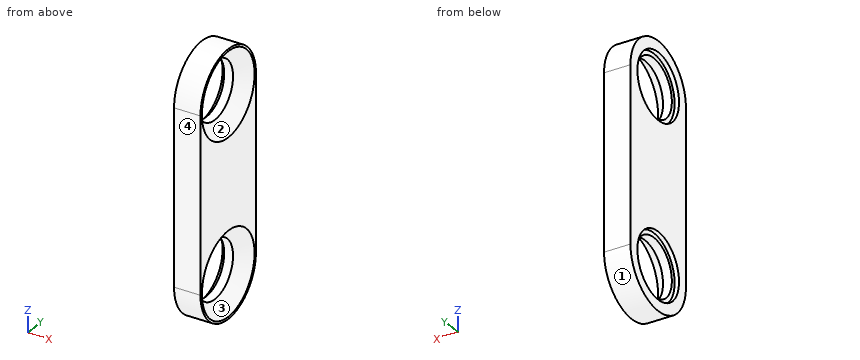
Autodesk Inventor part; units mm, degrees
ref_plane "YZ Plane" through (0, 0, 0) normal (1, 0, 0) x (0, 1, 0)
ref_plane "XZ Plane" through (0, 0, 0) normal (0, 1, 0) x (-1, 0, 0)
ref_plane "XY Plane" through (0, 0, 0) normal (0, 0, 1) x (1, 0, 0)
sketch "Boceto1" plane through (0, 0, 0) normal (1, 0, 0) x (0, 1, 0)
  line L0 (0, 0) -> (0, 19.75)
  circle A0 centre (0, 19.75) radius 5
  circle A1 centre (0, 0) radius 5
  line L1 (5, 0) -> (5, 19.75)
  line L2 (-5, 0) -> (-5, 19.75)
  circle A2 centre (0, 19.75) radius 3.25
  circle A3 centre (0, 0) radius 3.25
  dimension "d0" = 19.75
  dimension "d1" = 10
  dimension "d2" = 10
  dimension "d5" = 6.5
  dimension "d6" = 6.5
extrude "Extrusión1" add sketch "Boceto1" along normal mid plane 3
sketch "Boceto2" plane through (-1.5, 0, 0) normal (-1, 0, 0) x (0, 0, 1)
  circle A0 centre (0, 0) radius 3.75
  line L0 (0, 0) -> (19.75, 0)
  circle A1 centre (19.75, 0) radius 3.75
  dimension "d7" = 7.5
  dimension "d8" = 19.75
  dimension "d9" = 7.5
extrude "Extrusión2" cut sketch "Boceto2" against normal blind 0.5
chamfer "Chaflán1" distance 1.5 angle 45 2 edges at (1.5, -3.25, 19.75) (1.5, -3.25, 0)
equation "\"d0\" = m2_r3"
equation "\"d1\" = width_r3"
equation "\"d2\" = width_r3"
equation "\"d5\" = sj_diam_shaft + 0.5 * offset"
equation "\"d6\" = sj_diam_shaft + 0.5 * offset"
equation "\"d3\" = t_thikness"
equation "\"d7\" = sj_head_D + 0.5 * offset"
equation "\"d8\" = m2_r3"
equation "\"d9\" = sj_head_D + 0.5 * offset"
equation "\"d10\" = 0.5 * offset"
equation "\"offset\" = 1"
equation "\"m2_r3\" = 19.75"
equation "\"width_r3\" = 10"
equation "\"t_thikness\" = 3"
equation "\"sj_diam_shaft\" = 6"
equation "\"sj_head_D\" = 7"
equation "\"thikness\" = 2"
equation "\"r1\" = 5.55"
equation "\"r2o\" = 59.75"
equation "\"delta_y\" = 6"
equation "\"wire_d\" = 1"
equation "\"width_ang_spring\" = 5"
equation "\"spring_int_diam\" = 8.5"
equation "\"spring_ext_diam\" = 10.5"
equation "\"r3\" = 8.25"
equation "\"r3R\" = 4.75"
equation "\"r3T\" = 6.74537"
equation "\"alpha\" = 54.847297deg"
equation "\"alpha2\" = 270deg"
equation "\"theta3_recogido\" = 305.152703deg"
equation "\"delta_theta_3\" = 45deg"
equation "\"joint_width\" = 12"
equation "\"joint_radius\" = 7.75"
equation "\"shaft_width\" = 15"
equation "\"shaft_joint_diameter\" = 7.75"
equation "\"separation_space\" = 0.5"
equation "\"height_finger\" = 42"
equation "\"cell_screw_head_diameter\" = 4"
equation "\"cell_screw_diameter\" = 2"
equation "\"cell_space\" = 2"
equation "\"cell_width\" = 6"
equation "\"cell_theta_position\" = 60deg"
equation "\"cell_thikness\" = 1"
equation "\"cell_lenght\" = 37"
equation "\"cell_z_space\" = 5"
equation "\"wire_D\" = 2.3"
equation "\"width_link\" = 8"
equation "\"Dt\" = 1.05949"
equation "\"Djoint_shaft\" = 2.3"
equation "\"shaft_x\" = 1.45"
equation "\"shaft_y\" = 6.45"
equation "\"lenght_body_link\" = 186.05"
equation "\"lenght_bar_support\" = 201.65"
equation "\"wire_spring_d\" = 1"
equation "\"spring_int_d\" = 6"
equation "\"spring_lenght\" = 28"
equation "\"trigger_offset\" = 2"
equation "\"m2_theta2o\" = 107deg"
equation "\"m2_r2\" = 28"
equation "\"e\" = 9"
equation "\"So\" = 17"
equation "\"m2_theta3o\" = -30deg"
equation "\"m2_delta_theta1\" = 15deg"
equation "\"m2_theta3f\" = -60deg"
equation "\"trigger_thumb_lenght\" = 6"
equation "\"width_r12\" = 8"
equation "\"m2_r1\" = 25.2"
equation "\"r3_thikness\" = 3.5"
equation "\"tg_width\" = 4"
equation "\"pivot_screw_d\" = 4"
equation "\"pivot_diameter\" = 7"
equation "\"sj_groove\" = 2"
equation "\"sj_groove_deep\" = 7"
equation "\"sj_head_d\" = 4.7464"
equation "\"sj_head_height\" = 5"
equation "\"sf_lenght\" = 9.5"
equation "\"sf_base\" = 3"
equation "\"sf_head_height\" = 3"
equation "\"sf_head_width\" = 4.5"
equation "\"sf_head_offset\" = 0.25"
equation "\"sf_head_grip_width\" = 2"
equation "\"sf_head_angle\" = 45deg"
equation "\"sf_thikness\" = 5"
equation "\"screw_Dhead\" = 8"
equation "\"screw_d\" = 4"
equation "\"screw_lenght\" = 12"
equation "\"screwJ_base_D\" = 9"
equation "\"screwJ_top_D\" = 13"
equation "\"gj_D\" = 6"
equation "\"gj_d\" = 4"
equation "\"gj_out_section\" = 6"
equation "\"ext_width_slider\" = 3.5"
equation "\"sfbox_tip_width\" = 2.5"
equation "\"slim_width_slider\" = 1.5"
equation "\"agarradera_width\" = 4"
equation "\"int_width_slider\" = 2"
equation "\"agarradera_position\" = 82.13077"
equation "\"sfbox_theta1\" = 60deg"
equation "\"sfbox_theta2\" = 45deg"
equation "\"agarradera_theta\" = 60deg"
equation "\"sfbox_width\" = 1.5"
equation "\"box_fat_slider_lenght\" = 67"
equation "\"fat_width_slider\" = 2"
equation "\"box_in_width\" = 72"
equation "\"flex_separation_theta\" = 60deg"
equation "\"sf_flex_separation\" = 38.66667"
equation "\"thikness_box\" = 1.5"
equation "\"box_slim_slider_lenght\" = 116"
equation "\"box_in_deep\" = 77"
equation "\"box_in_height\" = 35"
properties part number "link3" material "Plástico PPS"
The model under review builds one solid part; all positions refer to its coordinate system, in mm. Face numbers are marked on the shaded views. Coordinates: 2 decimals unless noted, no trailing zeros. Order: outer loops, then holes, each group sorted by start corner. A loop starts at its lowest first (then second) coordinate and runs counter-clockwise, first axis right, second up. Notation, with made-up numbers: (-31, 46) -> (-6, 46) arc R30 ccw to (-6, 72) -> close; hole circle Ø4 at (32, 55). An arc over 180 degrees is marked (long way). Answer in a Markdown table with one row per item. Add a question column.
Item 1: Mouldability with a two-part tool opening along Y and no side actions: class the marked faces 1, 2, 3 and 4 as +Y half, -Y half, draft (parallel to the pull), parting line (faces both ways), or undercut.
Item 2: We need section C-C on y = -2.25. Give the number of separate pieces and of enclosed holes in the cut face, plus the area to 3 significant figures.
Item 3: We need section B-B on x = 0.65. Write out the cut boundary in (y, z).
Item 4: We need section A-A on y = 0. Write out the cut boundary in (x, z).
Item 5: Clearance check with flat-ended pins moving along their axes: pin 1 (1 mm diameter, centred on x = 0.5, y = -2.5, fed in from -Z); pin 2 (1 mm diameter, centred on y = -3, z = 18, fed in from +X). State where each tip first meets the part, or that it passes through.
Item 6: To check wall thickness, follow probe 1 along Z at (x, y) = (-0.25, 0); probe 2 along Z at (x, y) = (-0.4, 0.75); probe 3 along Y at (x, z) = (-1.35, 0). State the ranges of each line that lie inside material, in increasing order.
Final values:
| question | item | result |
|---|---|---|
| 1 | face 1 | parting line |
| 1 | face 2 | undercut |
| 1 | face 3 | undercut |
| 1 | face 4 | -Y half |
| 2 | separate pieces | 3 |
| 2 | enclosed holes | 0 |
| 2 | area | 50.9 mm2 |
| 3 | outline | (-5, 0) arc R5 ccw to (5, 0) -> (5, 19.75) arc R5 ccw to (-5, 19.75) -> close; hole circle Ø7.8 at (0, 0); hole circle Ø7.8 at (0, 19.75) |
| 4 | outline | (-1.5, -5) -> (1.5, -5) -> (1.5, -4.75) -> (0, -3.25) -> (-1, -3.25) -> (-1, -3.75) -> (-1.5, -3.75) -> close; (-1.5, 3.75) -> (-1, 3.75) -> (-1, 3.25) -> (0, 3.25) -> (1.5, 4.75) -> (1.5, 15) -> (0, 16.5) -> (-1, 16.5) -> (-1, 16) -> (-1.5, 16) -> close; (-1.5, 23.5) -> (-1, 23.5) -> (-1, 23) -> (0, 23) -> (1.5, 24.5) -> (1.5, 24.75) -> (-1.5, 24.75) -> close |
| 5 | pin 1 | stops at z = -4.58 |
| 5 | pin 2 | stops at x = 0.72 |
| 6 | probe 1 | z = -5 to -3.25, 3.25 to 16.5, 23 to 24.75 |
| 6 | probe 2 | z = -4.94 to -3.16, 3.16 to 16.59, 22.91 to 24.69 |
| 6 | probe 3 | y = -5 to -3.75, 3.75 to 5 |
